```python
from build123d import *

# Parameters (mm, degrees)
SKETCH_W        = 40
SKETCH_H        = 13.5
PAD_DEPTH       = 1.5
FILLET_R        = 2
SKETCH001_R     = 0.8
POCKET_DEPTH    = 5
SKETCH002_R     = 4
PAD001_DEPTH    = 2.5
SKETCH003_R     = 1.5
POCKET001_DEPTH = 1
SKETCH004_R     = 3
POCKET002_DEPTH = 3


with BuildPart() as part:
    # Sketch → Pad (new body)
    with BuildSketch(Plane.XY):
        Rectangle(SKETCH_W, SKETCH_H)
    extrude(amount=PAD_DEPTH)

    # Fillet
    fillet_edges = [part.edges().sort_by_distance(p)[0] for p in [
        (-20, -6.75, 0.75),
        (-20, 6.75, 0.75),
        (20, 6.75, 0.75),
        (20, -6.75, 0.75),
    ]]
    fillet(fillet_edges, radius=FILLET_R)

    # Sketch001 (on Face5 of Fillet) → Pocket (cut)
    with BuildSketch(Plane.XY.offset(1.5)):
        with Locations((-11, 5.75)):
            Circle(SKETCH001_R)
    pocket = extrude(amount=-POCKET_DEPTH, mode=Mode.SUBTRACT)

    # Mirrored: Pocket across Sketch001 V_Axis
    add(pocket.mirror(Plane(origin=(0, 0, 1.5), x_dir=(0, 0, 1), z_dir=(1, 0, 0))), mode=Mode.SUBTRACT)

    # Sketch002 (on Face5 of Mirrored) → Pad001 (join)
    with BuildSketch(Plane.XY.offset(1.5)):
        with Locations((-12.5, 0)):
            Circle(SKETCH002_R)
    pad001 = extrude(amount=PAD001_DEPTH)

    # Mirrored001: Pad001 across Sketch002 V_Axis
    add(pad001.mirror(Plane(origin=(0, 0, 1.5), x_dir=(0, 0, 1), z_dir=(1, 0, 0))))

    # Sketch003 (on Face15 of Mirrored001) → Pocket001 (cut)
    with BuildSketch(Plane.XY.offset(4)):
        with Locations((-12.5, 0)):
            Circle(SKETCH003_R)
    pocket001 = extrude(amount=-POCKET001_DEPTH, mode=Mode.SUBTRACT)

    # Mirrored002: Pocket001 across Sketch003 V_Axis
    add(pocket001.mirror(Plane(origin=(0, 0, 4), x_dir=(0, 0, 1), z_dir=(1, 0, 0))), mode=Mode.SUBTRACT)

    # Sketch004 (on Face2 of Mirrored002) → Pocket002 (cut)
    with BuildSketch(Plane(origin=(0, 0, 0), x_dir=(1, 0, 0), z_dir=(0, 0, -1))):
        with Locations((-12.5, 0)):
            Circle(SKETCH004_R)
    pocket002 = extrude(amount=-POCKET002_DEPTH, mode=Mode.SUBTRACT)

    # Mirrored003: Pocket002 across Sketch004 V_Axis
    add(pocket002.mirror(Plane(origin=(0, 0, 0), x_dir=(0, 0, -1), z_dir=(1, 0, 0))), mode=Mode.SUBTRACT)


solid = part.part
```
CAD build for the part. Positions are in the model's coordinates, mm. A direction names the side the tool comes from. Round coordinates to 2 decimals unless told otherwise and drop trailing zeros. Write each loop counter-clockwise with the first axis right and the second up, starting at its lowest first coordinate (ties: lowest second). Pieces come first, ordered by that corner, then holes.
Item 1: Drop flat-ended pins along their axis: pin 1 Ø5.5 at (x, y) = (-12.5, 0) entering from -Z; pin 2 Ø3 at (x, y) = (3.5, -5.5) entering from +Z. Give the stop position or say it passes through.
Filled in:
pin 1: stops at z = 3
pin 2: stops at z = 1.5
Item 2: Mould opens along Y. For faces 1 (the cylindrical face through (14.9, 1.8, 1.5)), 2 (the flat face through (0, -6.75, 1)), 3 (the flat face through (-20, 0, 1)) say: released by +Y, released by -Y, zero draft, split by the parting line, or undercut.
Filled in:
face 1: undercut
face 2: released by -Y
face 3: zero draft
Item 3: Band-saw the part on B-B on z = 3.4. Write the cut outline in (x, y), then the cut area to 3 significant figures.
Filled in:
outline: circle Ø8 at (-12.5, 0); circle Ø8 at (12.5, 0); hole circle Ø3 at (-12.5, 0); hole circle Ø3 at (12.5, 0)
area: 86.4 mm2
Item 4: Band-saw the part on D-D on x = 0. Write the cut outline in (y, z), then the cut area to 4 significant figures.
Filled in:
outline: (-6.75, 0) - (6.75, 0) - (6.75, 1.5) - (-6.75, 1.5) - close
area: 20.25 mm2
Item 5: Tool access for faces 4 (the cylindrical face through (15.7, -2.4, 2.7)), 5 (the cylindrical face through (-14.9, 1.8, 1.5)), 6 (the flat face through (0, 0, 0)): list every direction of +Z, -Z, +X, -X, +Y, -Y with a clear straight run to the whole face (end or side of a thin tool).
Filled in:
face 4: +Z
face 5: -Z
face 6: -Z, +X, -X, +Y, -Y
Item 6: Band-saw the part on A-A on x = -12.5. Write the cut outline in (y, z).
Filled in:
outline: (-6.75, 0) - (-3, 0) - (-3, 3) - (-1.5, 3) - (-1.5, 4) - (-4, 4) - (-4, 1.5) - (-6.75, 1.5) - close; (1.5, 3) - (3, 3) - (3, 0) - (6.75, 0) - (6.75, 1.5) - (4, 1.5) - (4, 4) - (1.5, 4) - close
Item 7: Drill centre lines: L1, parallel to X at y = 0, z = 1.3; L2, parallel to X at y = -0.5, z = 1.7; L3, parallel to X at y = -1.25, z = 3.6. Where is each one in solid material? Low to high.
Filled in:
L1: x = -20 to -15.5, -9.5 to 9.5, 15.5 to 20
L2: x = -16.47 to -15.46, -9.54 to -8.53, 8.53 to 9.54, 15.46 to 16.47
L3: x = -16.3 to -13.33, -11.67 to -8.7, 8.7 to 11.67, 13.33 to 16.3
Item 8: Band-saw the part on C-C on y = -0.75. Write the cut outline in (x, z), then the cut area to 3 significant figures.
Filled in:
outline: (-20, 0) - (-15.4, 0) - (-15.4, 3) - (-13.8, 3) - (-13.8, 4) - (-16.43, 4) - (-16.43, 1.5) - (-20, 1.5) - close; (-11.2, 3) - (-9.6, 3) - (-9.6, 0) - (9.6, 0) - (9.6, 3) - (11.2, 3) - (11.2, 4) - (8.57, 4) - (8.57, 1.5) - (-8.57, 1.5) - (-8.57, 4) - (-11.2, 4) - close; (13.8, 3) - (15.4, 3) - (15.4, 0) - (20, 0) - (20, 1.5) - (16.43, 1.5) - (16.43, 4) - (13.8, 4) - close
area: 59.2 mm2
